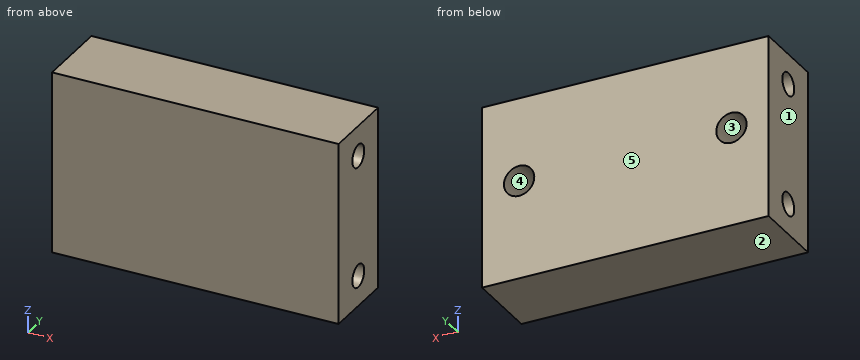
```python
from build123d import *

# Parameters (mm, degrees)
SKETCH_1_W                  = 37.8
SKETCH_1_H                  = 24
EXTRUDE_1_DEPTH             = 10
HOLE_WIZARD_M4_1_AT_2_COUNT = 2
HOLE_WIZARD_M4_1_AT_2_PITCH = 28
HOLE_WIZARD_M3_1_AT_2_COUNT = 2
HOLE_WIZARD_M3_1_AT_2_PITCH = 16


with BuildPart() as part:
    # 草图1 → 凸台-拉伸1 (new body)
    with BuildSketch(Plane(origin=(0, 0, 0), x_dir=(1, 0, 0), z_dir=(0, 1, 0))):
        Rectangle(SKETCH_1_W, SKETCH_1_H)
    extrude(amount=EXTRUDE_1_DEPTH)

    # 草图5 → M4 螺纹孔1 (revolve, cut)
    with BuildSketch(Plane(origin=(-14, 10, 1), x_dir=(0, 0, 1), z_dir=(1, 0, 0))):
        Polygon((0, 0), (0, 8.491420021), (1.65, 7.5), (1.65, 8), (2, 8), (2, 0), align=None)
    hole_wizard_m4_1 = revolve(axis=Axis((-14, 16.35, 1), (0, -1, 0)), mode=Mode.SUBTRACT)

    # M4 螺纹孔1 at 2: M4 螺纹孔1 ×2
    with Locations(*[(i * HOLE_WIZARD_M4_1_AT_2_PITCH, 0, 0) for i in range(1, HOLE_WIZARD_M4_1_AT_2_COUNT)]):
        add(hole_wizard_m4_1, mode=Mode.SUBTRACT)

    # 草图6 → M3 螺纹孔1 (revolve, cut)
    with BuildSketch(Plane(origin=(18.9, 5, 8), x_dir=(0, 0, -1), z_dir=(0, 1, 0))):
        Polygon((0, 0), (0, 12.751075774), (1.25, 12), (1.25, 11.5), (1.5, 11.5), (1.5, 0), align=None)
    hole_wizard_m3_1 = revolve(axis=Axis((25.25, 5, 8), (-1, 0, 0)), mode=Mode.SUBTRACT)

    # M3 螺纹孔1 at 2: M3 螺纹孔1 ×2
    with Locations(*[(0, 0, -i * HOLE_WIZARD_M3_1_AT_2_PITCH) for i in range(1, HOLE_WIZARD_M3_1_AT_2_COUNT)]):
        add(hole_wizard_m3_1, mode=Mode.SUBTRACT)

    # 镜向1: M3 螺纹孔1 across plane
    add(hole_wizard_m3_1.mirror(Plane(origin=(0, 0, 0), x_dir=(0, 0, 1), z_dir=(1, 0, 0))), mode=Mode.SUBTRACT)

    # 镜向1 copy 1 sketch → 镜向1 copy 1 (revolve, cut)
    with BuildSketch(Plane(origin=(-18.9, 5, -8), x_dir=(0, 0, -1), z_dir=(0, 1, 0))):
        Polygon((0, 0), (0, -12.751075774), (1.25, -12), (1.25, -11.5), (1.5, -11.5), (1.5, 0), align=None)
    revolve(axis=Axis((-25.25, 5, -8), (-1, 0, 0)), mode=Mode.SUBTRACT)


solid = part.part
```
Model file for the job. Use its own axes, mm. Face numbers are marked on the shaded views. A direction names the side the tool comes from. Coordinates: 2 decimals unless noted, no trailing zeros. Loops run counter-clockwise (first coordinate to the right, second up) from the corner with the lowest first, then second, coordinate; pieces in that order, holes last. Notation, with made-up numbers: (68.5, -2.75) -> (73.5, -2.75) arc R33 cw to (73.5, 27.25) -> close; hole circle Ø2 at (59, 10). An arc over 180 degrees is marked (long way). Answer as a JSON object with one key per item and string values.
Q1. Pull direction X, two halves, no side cores. Call the marked faces 1, 2 and 3: released by +X, released by -X, zero draft, split by the parting line, or undercut.
Report:
{"face 1": "released by -X", "face 2": "zero draft", "face 3": "undercut"}
Q2. 3-axis set-ups, long thin cutter, end or side, ignore diameter. For the marked faces 4 and 5: which of +Z, -Z, +X, -X, +Y, -Y reach the whole face in a straight line?
Report:
{"face 4": "+Y", "face 5": "+Z, -Z, +X, -X, +Y"}
Q3. Cut at A-A (x = 10.5). List the corners of the cut face in (y, z).
Report:
{"outline": "(0, -12) -> (10, -12) -> (10, 12) -> (0, 12) -> close; hole circle Ø3 at (5, -8); hole circle Ø3 at (5, 8)"}
Q4. Probe probe 1 along Z at (x, y) = (-7.15, 5); probe 2 along Z at (x, y) = (10.25, 5); probe 3 along Y at (x, z) = (-13, -8). List the from-to ranges inside material, lowest first.
Report:
{"probe 1": "z = -12 to -9.25, -6.75 to 6.75, 9.25 to 12", "probe 2": "z = -12 to -9.5, -6.5 to 6.5, 9.5 to 12", "probe 3": "y = 0 to 3.5, 6.5 to 10"}
Q5. Cut at B-B (y = 7.75). List the corners of the cut face in (x, z).
Report:
{"outline": "(-18.9, -12) -> (18.9, -12) -> (18.9, 12) -> (-18.9, 12) -> close; hole circle Ø4 at (-14, 1); hole circle Ø4 at (14, 1)"}
Q6. Flat gauge pins, fed straight in: P1, Ø2, axis at y = 5, z = 8, coming from the -X side; P2, Ø0.9, axis at y = 4.5, z = 7.5, coming from the +X side; P3, Ø1.8, axis at y = 5, z = -8, coming from the -X side. Where does each tip first touch, or does it go through?
Report:
{"P1": "stops at x = -6.75", "P2": "stops at x = 6.84", "P3": "stops at x = -6.69"}
